Model file for the job. Use its own axes, mm. Face numbers are marked on the shaded views. A direction names the side the tool comes from. Coordinates: 2 decimals unless noted, no trailing zeros. Order: outer loops, then holes, each group sorted by start corner. A loop starts at its lowest first (then second) coordinate and runs counter-clockwise, first axis right, second up. Notation, with made-up numbers: (2.25, 11) -> (15.25, 11) arc R9 cw to (15.25, 20) -> close; hole circle Ø4 at (86.5, 79). An arc over 180 degrees is marked (long way). Write item = value, one per line. Start each with the question number.
Q1. Cut at D-D, the plane y = -17.5. List the corners of the cut face in (x, z).
Q2. Cut at B-B, the plane y = 27.5. List the corners of the cut face in (x, z), plus the area to 3 significant figures.
Q3. Mould opens along X. For the marked faces 1, 2, 3 and 4 say: +X half, -X half, draft (parallel to the pull), parting line (faces both ways), or undercut.
Q4. Cut at C-C, the plane z = -54. List the corners of the cut face in (x, y), plus the area to 3 significant figures.
Q5. Wall check: line 1 (Y direction, x = -20, z = -38.5); line 2 (X direction, y = 17.5, z = 2); line 3 (Y direction, x = 0, z = -21). Give the ranges that are in metal, low to high. Write a range as from..to.
Q6. Flat gauge pins, fed straight in: pin 1 (3.5 mm diameter, centred on x = -30.31, y = 17.5, fed in from -Z); pin 2 (8 mm diameter, centred on x = -30.31, y = -17.5, fed in from -Z); pin 3 (12 mm diameter, centred on x = 23, z = -62, fed in from -Y); pin 4 (1.5 mm diameter, centred on y = -29.5, z = -7, fed in from +X). Where does each tip first touch, or does it go through?
Q7. Cut at A-A, the plane y = 0. List the corners of the cut face in (x, z).
Q8. 3-axis set-ups, long thin cutter, end or side, ignore diameter. For the marked faces 5, 6 and 7: which of +Z, -Z, +X, -X, +Y, -Y reach the whole face in a straight line?
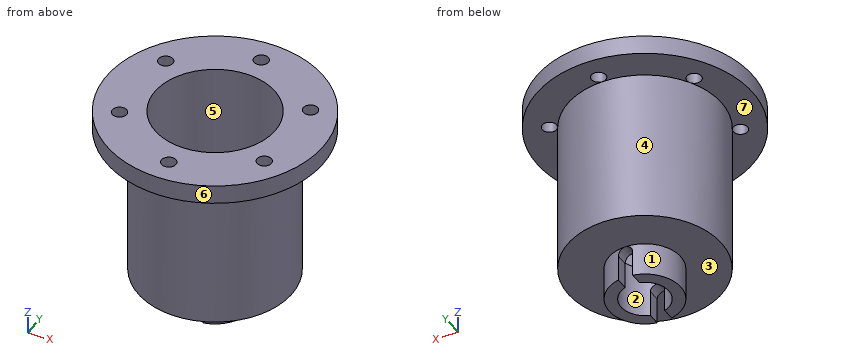
from build123d import *

# Parameters (mm, degrees)
SZKIC1_R                        = 45
SZKIC1_R_2                      = 3
DODANIE_WYCI_GNI_CIE1_DEPTH     = 8
SZKIC2_R                        = 32
DODANIE_WYCI_GNI_CIE2_DEPTH     = 65
SZKIC3_R                        = 15
DODANIE_WYCI_GNI_CIE3_DEPTH     = 14
SZKIC4_R                        = 10
WYTNIJ_WYCI_GNI_CIE1_DEPTH      = 96
SZKIC5_R                        = 25
WYTNIJ_WYCI_GNI_CIE2_DEPTH      = 65
WYTNIJ_WYCI_GNI_CIE3_DEPTH      = 19
WYTNIJ_WYCI_GNI_CIE3_DEPTH_BACK = 19


with BuildPart() as part:
    # Szkic1 → Dodanie-wyci_gni_cie1 (new body)
    with BuildSketch(Plane.XY):
        Circle(SZKIC1_R)
        with Locations((0, 35)):
            Circle(SZKIC1_R_2, mode=Mode.SUBTRACT)
        with Locations((-30.310889132, 17.5)):
            Circle(SZKIC1_R_2, mode=Mode.SUBTRACT)
        with Locations((30.310889132, -17.5)):
            Circle(SZKIC1_R_2, mode=Mode.SUBTRACT)
        with Locations((30.310889132, 17.5)):
            Circle(SZKIC1_R_2, mode=Mode.SUBTRACT)
        with Locations((-30.310889132, -17.5)):
            Circle(SZKIC1_R_2, mode=Mode.SUBTRACT)
        with Locations((0, -35)):
            Circle(SZKIC1_R_2, mode=Mode.SUBTRACT)
    extrude(amount=DODANIE_WYCI_GNI_CIE1_DEPTH)

    # Szkic2 → Dodanie-wyci_gni_cie2 (add)
    with BuildSketch(Plane(origin=(0, 0, 0), x_dir=(-1, 0, 0), z_dir=(0, 0, -1))):
        Circle(SZKIC2_R)
    extrude(amount=DODANIE_WYCI_GNI_CIE2_DEPTH)

    # Szkic3 → Dodanie-wyci_gni_cie3 (add)
    with BuildSketch(Plane(origin=(0, 0, -65), x_dir=(-1, 0, 0), z_dir=(0, 0, -1))):
        Circle(SZKIC3_R)
    extrude(amount=DODANIE_WYCI_GNI_CIE3_DEPTH)

    # Szkic4 → Wytnij-wyci_gni_cie1 (cut)
    with BuildSketch(Plane(origin=(0, 0, -79), x_dir=(-1, 0, 0), z_dir=(0, 0, -1))):
        Circle(SZKIC4_R)
    extrude(amount=-WYTNIJ_WYCI_GNI_CIE1_DEPTH, mode=Mode.SUBTRACT)

    # Szkic5 → Wytnij-wyci_gni_cie2 (cut)
    with BuildSketch(Plane.XY.offset(8)):
        Circle(SZKIC5_R)
    extrude(amount=-WYTNIJ_WYCI_GNI_CIE2_DEPTH, mode=Mode.SUBTRACT)

    # Szkic6 → Wytnij-wyci_gni_cie3 (cut, two sides)
    with BuildSketch(Plane(origin=(0, 0, 0), x_dir=(1, 0, 0), z_dir=(0, 1, 0))) as wytnij_wyci_gni_cie3_sk:
        with BuildLine():
            Line((-3, 85.590042605), (3, 85.590042605))
            Line((3, 85.590042605), (3, 68))
            ThreePointArc((3, 68), (0, 65), (-3, 68))
            Line((-3, 68), (-3, 85.590042605))
        make_face()
    extrude(amount=WYTNIJ_WYCI_GNI_CIE3_DEPTH, mode=Mode.SUBTRACT)
    extrude(wytnij_wyci_gni_cie3_sk.sketch, amount=-WYTNIJ_WYCI_GNI_CIE3_DEPTH_BACK, mode=Mode.SUBTRACT)


solid = part.part
Here are the results:
q1.outline = (-41.46, 0) -> (-33.31, 0) -> (-33.31, 8) -> (-41.46, 8) -> close; (-27.31, 0) -> (-26.79, 0) -> (-26.79, -65) -> (26.79, -65) -> (26.79, 0) -> (27.31, 0) -> (27.31, 8) -> (17.85, 8) -> (17.85, -57) -> (-17.85, -57) -> (-17.85, 8) -> (-27.31, 8) -> close; (33.31, 0) -> (41.46, 0) -> (41.46, 8) -> (33.31, 8) -> close
q2.outline = (-35.62, 0) -> (-16.36, 0) -> (-16.36, -65) -> (16.36, -65) -> (16.36, 0) -> (35.62, 0) -> (35.62, 8) -> (-35.62, 8) -> close
q2.area = 2,700 mm²
q3.face_1 = -X half
q3.face_2 = undercut
q3.face_3 = draft
q3.face_4 = parting line
q4.outline = circle Ø64 at (0, 0); hole circle Ø50 at (0, 0)
q4.area = 1,250 mm²
q5.line_1 = -24.98..-15, 15..24.98
q5.line_2 = -41.46..-33.31, -27.31..-17.85, 17.85..27.31, 33.31..41.46
q5.line_3 = -32..-25, 25..32
q6.pin_1 = through
q6.pin_2 = -65
q6.pin_3 = -27.11
q6.pin_4 = 14.05
q7.outline = (-45, 0) -> (-32, 0) -> (-32, -65) -> (-15, -65) -> (-15, -79) -> (-10, -79) -> (-10, -57) -> (-25, -57) -> (-25, 8) -> (-45, 8) -> close; (10, -79) -> (15, -79) -> (15, -65) -> (32, -65) -> (32, 0) -> (45, 0) -> (45, 8) -> (25, 8) -> (25, -57) -> (10, -57) -> close
q8.face_5 = +Z
q8.face_6 = +Z, -Z
q8.face_7 = -Z
